Work out the finished part from the listing and answer in its coordinate system (mm). Face numbers are marked on the shaded views. A direction names the side the tool comes from. Give positions to 0.01 mm unless a question says otherwise; leave off trailing zeros. Loops run counter-clockwise (first coordinate to the right, second up) from the corner with the lowest first, then second, coordinate; pieces in that order, holes last.
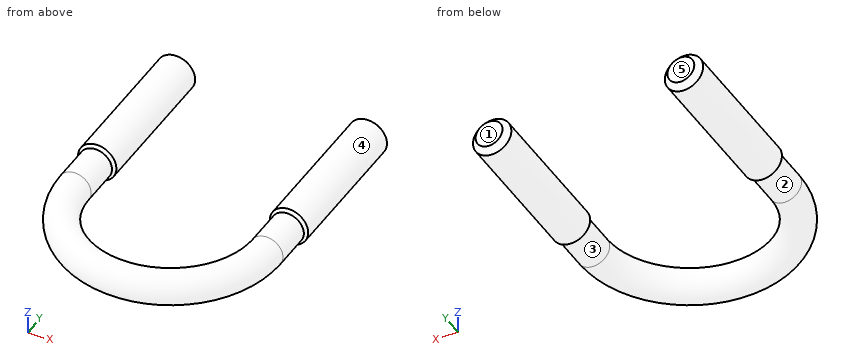
from build123d import *

# Parameters (mm, degrees)
SKETCH2_R           = 3.175
BOSS_EXTRUDE1_DEPTH = 25.4
CHAMFER2_SIZE       = 0.9525
CHAMFER3_SIZE       = 0.4699
SKETCH12_R          = 2.7051
SKETCH9_R           = 3.175
BOSS_EXTRUDE2_DEPTH = 2.778125
SKETCH10_OUTSIDE_W  = 233.937
SKETCH10_OUTSIDE_H  = 203.708
SKETCH10_OUTSIDE_R  = 5.55625
CUT_EXTRUDE1_DEPTH  = 51.205782884
CUT_EXTRUDE1_DRAFT  = -60
SKETCH11_OUTSIDE_W  = 217.071
SKETCH11_OUTSIDE_H  = 186.842
SKETCH11_OUTSIDE_R  = 5.55625
CUT_EXTRUDE2_DEPTH  = 46.336665415
CUT_EXTRUDE2_DRAFT  = -60
CHAMFER4_SIZE       = 0.381
LPATTERN1_COUNT     = 2
LPATTERN1_PITCH     = 31.75


with BuildPart() as part:
    # Sketch2 → Boss-Extrude1 (new body)
    with BuildSketch(Plane(origin=(0, 31.75, 0), x_dir=(-1, 0, 0), z_dir=(0, 1, 0))):
        with Locations(Location((15.875, 0, 0), (0, 0, 90))):
            Circle(SKETCH2_R)
    extrude(amount=-BOSS_EXTRUDE1_DEPTH)

    # Chamfer2
    chamfer2_edges = [part.edges().sort_by_distance(p)[0] for p in [
        (-15.875, 31.75, -3.175),
    ]]
    chamfer(chamfer2_edges, length=CHAMFER2_SIZE)

    # Chamfer3
    chamfer3_edges = [part.edges().sort_by_distance(p)[0] for p in [
        (-15.875, 6.35, -3.175),
    ]]
    chamfer(chamfer3_edges, length=CHAMFER3_SIZE)


with BuildPart() as body_2:
    # Mirror2: mirrored copy
    add(part.part.mirror(Plane(origin=(0, 0, 0), x_dir=(0, 0, 1), z_dir=(1, 0, 0))))


with BuildPart() as part_1:
    add(part.part)

    add(body_2.part)  # Sweep1 merges body 2
    # Sweep1: sweep along a path in Sketch8
    with BuildLine(Plane.XY) as sweep1_path:
        Line((-15.875, 19.05), (-15.875, 0))
        ThreePointArc((-15.875, 0), (0, -15.875), (15.875, 0))
        Line((15.875, 0), (15.875, 19.05))
    # Sketch12 → Sweep1 (sweep)
    with BuildSketch(Plane(origin=(0, 0, 0), x_dir=(0, 0, -1), z_dir=(1, 0, 0))):
        with Locations((0, -15.875)):
            Circle(SKETCH12_R)
    sweep(path=sweep1_path.line)


with BuildPart() as body_2_2:
    # Sketch9 → Boss-Extrude2 (new, symmetric)
    with BuildSketch(Plane(origin=(0, 23.283333333, 0), x_dir=(-1, 0, 0), z_dir=(0, 1, 0))):
        Polygon((-19.082902433, 5.55625), (-22.290804866, 0), (-19.082902433, -5.55625), (-12.667097567, -5.55625), (-9.459195134, 0), (-12.667097567, 5.55625), align=None)
        with Locations(Location((-15.875, 0, 0), (0, 0, 90))):
            Circle(SKETCH9_R, mode=Mode.SUBTRACT)
    extrude(amount=BOSS_EXTRUDE2_DEPTH, both=True)


with BuildPart() as cut_extrude1_tool:
    # Sketch10 outside → Cut-Extrude1 (with draft: the straight prism first)
    with BuildSketch(Plane(origin=(0, 26.061458333, 0), x_dir=(1, 0, 0), z_dir=(0, 1, 0))):
        with Locations((1.6205, 0)):
            Rectangle(SKETCH10_OUTSIDE_W, SKETCH10_OUTSIDE_H)
        with Locations((15.875, 0)):
            Circle(SKETCH10_OUTSIDE_R, mode=Mode.SUBTRACT)
    extrude(amount=-CUT_EXTRUDE1_DEPTH)
    # Cut-Extrude1: the draft: its side faces are tilted about the plane it starts from
    cut_extrude1_sides = [cut_extrude1_tool.faces().sort_by_distance(p)[0] for p in [
        (1.6205, 0.458566891, 101.854),
        (118.589, 0.458566891, 0),
        (1.6205, 0.458566891, -101.854),
        (-115.348, 0.458566891, 0),
        (10.31875, 0.458566891, 0),
    ]]
    draft(cut_extrude1_sides, Plane(origin=(0, 26.061458333, 0), x_dir=(1, 0, 0), z_dir=(0, 1, 0)), CUT_EXTRUDE1_DRAFT)


with BuildPart() as body_2_2_1:
    add(body_2_2.part)

    # Cut-Extrude1: cut by cut_extrude1_tool
    add(cut_extrude1_tool.part, mode=Mode.SUBTRACT)


with BuildPart() as cut_extrude2_tool:
    # Sketch11 outside → Cut-Extrude2 (with draft: the straight prism first)
    with BuildSketch(Plane.XZ.offset(-20.505208333)):
        with Locations((1.6205, 0)):
            Rectangle(SKETCH11_OUTSIDE_W, SKETCH11_OUTSIDE_H)
        with Locations((15.875, 0)):
            Circle(SKETCH11_OUTSIDE_R, mode=Mode.SUBTRACT)
    extrude(amount=-CUT_EXTRUDE2_DEPTH)
    # Cut-Extrude2: the draft: its side faces are tilted about the plane it starts from
    cut_extrude2_sides = [cut_extrude2_tool.faces().sort_by_distance(p)[0] for p in [
        (1.6205, 43.673541041, -93.421),
        (110.156, 43.673541041, 0),
        (1.6205, 43.673541041, 93.421),
        (-106.915, 43.673541041, 0),
        (10.31875, 43.673541041, 0),
    ]]
    draft(cut_extrude2_sides, Plane.XZ.offset(-20.505208333), CUT_EXTRUDE2_DRAFT)


with BuildPart() as body_2_2_2:
    add(body_2_2_1.part)

    # Cut-Extrude2: cut by cut_extrude2_tool
    add(cut_extrude2_tool.part, mode=Mode.SUBTRACT)

    # Chamfer4
    chamfer4_edges = [body_2_2_2.edges().sort_by_distance(p)[0] for p in [
        (15.875, 20.505208333, -3.175),
        (15.875, 26.061458333, -3.175),
    ]]
    chamfer(chamfer4_edges, length=CHAMFER4_SIZE)


with BuildPart() as lpattern1_1:
    # LPattern1: pattern copy
    add(body_2_2_2.part.moved(Location(Vector(-1, 0, 0) * (1 * LPATTERN1_PITCH))))


solid = part_1.part
Item 1: Find section A-A, the plane z = 0. Write down the section's boundary in (x, y).
Item 2: Find section C-C, the plane y = 1. Write down the section's boundary in (x, z) (3 decimals).
Item 3: Find section B-B, the plane y = 25. Write down the section's boundary in (x, z) (3 decimals), plus the area to 3 significant figures.
Item 4: Flat-ended cylindrical pins translate along their axes: pin 1 Ø1.5 at (x, y) = (-12.5, -8) entering from +Z; pin 2 Ø1.5 at (x, z) = (-9.5, 0) entering from -Y; pin 3 Ø8 at (x, y) = (13, 20) entering from -Z (3 decimals); pin 4 Ø4 at (x, y) = (-10.5, -12) entering from -Z. Find the tip coordinate at first contact, or state that the pin passes through.
Item 5: Determine the mould class of the marked faces 1 and 2 for opening direction X: released by +X, released by -X, zero draft, split by the parting line, or undercut.
Item 6: For the marked faces 3, 4 and 5, determine the directions among +Z, -Z, +X, -X, +Y, -Y from which every point of the face is accessible in a straight line to the end or side of a thin tool.
Item 7: Consider line 1 (X direction, y = 23, z = 0); line 2 (X direction, y = 29.5, z = -0.75); line 3 (Y direction, x = -14, z = 1). Determine where each line is inside the solid, lowest interval first.
Ans:
1. outline: (-19.05, 6.82) - (-18.58, 6.35) - (-18.58, 0) arc R18.58 ccw to (18.58, 0) - (18.58, 6.35) - (19.05, 6.82) - (19.05, 30.8) - (18.1, 31.75) - (13.65, 31.75) - (12.7, 30.8) - (12.7, 6.82) - (13.17, 6.35) - (13.17, 0) arc R13.17 cw to (-13.17, 0) - (-13.17, 6.35) - (-12.7, 6.82) - (-12.7, 30.8) - (-13.65, 31.75) - (-18.1, 31.75) - (-19.05, 30.8) - close
2. outline: circle Ø5.41 at (-15.875, 0); circle Ø5.41 at (15.875, 0)
3. outline: circle Ø6.35 at (-15.875, 0); circle Ø6.35 at (15.875, 0)
3. area: 63.3 mm2
4. pin 1: stops at z = 2.69
4. pin 2: stops at y = -16.39
4. pin 3: stops at z = -3.175
4. pin 4: stops at z = -2.71
5. face 1: zero draft
5. face 2: undercut
6. face 3: none
6. face 4: +Y
6. face 5: +Z, -Z, +X, -X, +Y
7. line 1: x = -19.05 to -12.7, 12.7 to 19.05
7. line 2: x = -18.96 to -12.79, 12.79 to 18.96
7. line 3: y = -11.92 to 31.75
